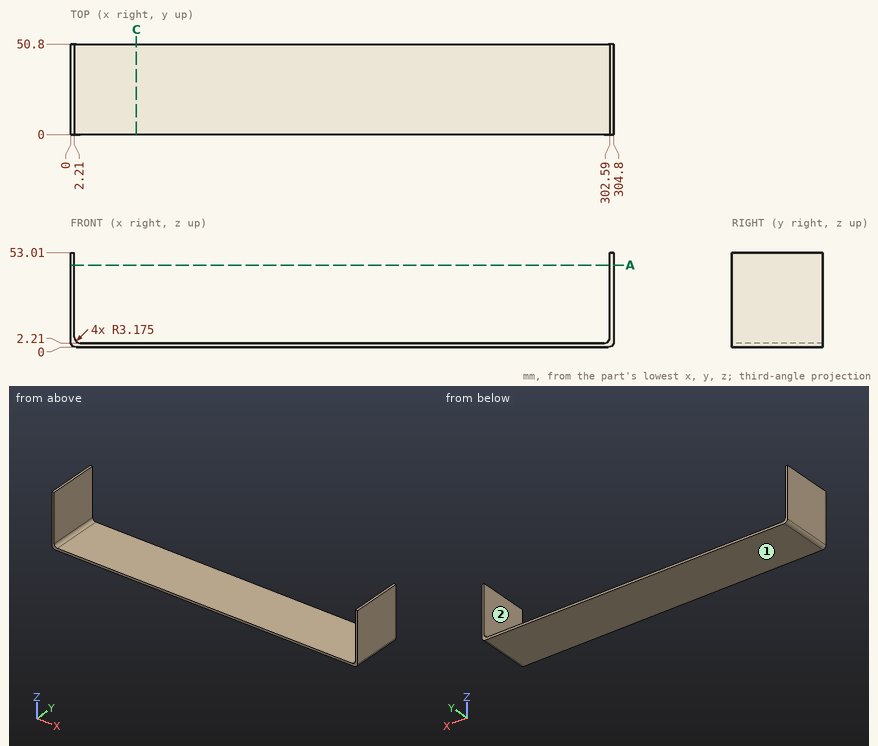
Geometry check sheet. Reference: drawing and pictorial views, mm from the part's lowest x, y, z. A direction names the side the tool comes from. Give positions to 0.01 mm unless a question says otherwise; leave off trailing zeros. Order: outer loops, then holes, each group sorted by start corner. A loop starts at its lowest first (then second) coordinate and runs counter-clockwise, first axis right, second up. Notation, with made-up numbers: M 75.25,26.25 L 111.25,26.25 A23 cw 111.25,61.25 Z; hole C 20,-9.75 d5. An arc over 180 degrees is marked long. Return JSON: item names as keys, results as strings. Group by question number.
1) Scan lines: line 1 (X direction, y = 6, z = 46.5); line 2 (Z direction, x = 145, y = 47); line 3 (X direction, y = 30.5, z = 3) (1 decimal). Record each from-to range of solid material in increasing order.
2) Go/stop test with a flat-tipped pin: pin 1 Ø12 at (x, y) = (234.5, 40.5) entering from +Z. Record where the tip stops, or that it passes through.
3) Section check A-A on z = 46. Record the cut outline in (x, y).
4) Access from +Z, -Z, +X, -X, +Y, -Y to the whole of each face (thin tool, end or side, straight path). Record for the marked faces 1 and 2.
5) Section check C-C on x = 37. Record the cut outline in (y, z).
Answer block:
{
 "1": {"line 1": "x = 0 to 2.21, 302.59 to 304.8", "line 2": "z = 0 to 2.21", "line 3": "x = 0 to 3.3, 301.5 to 304.8"},
 "2": {"pin 1": "stops at z = 2.21"},
 "3": {"outline": "M 0,0 L 2.21,0 L 2.21,50.8 L 0,50.8 Z; M 302.59,0 L 304.8,0 L 304.8,50.8 L 302.59,50.8 Z"},
 "4": {"face 1": "-Z, +X, -X, +Y, -Y", "face 2": "+Z, +Y, -Y"},
 "5": {"outline": "M 0,0 L 50.8,0 L 50.8,2.21 L 0,2.21 Z"}
}
